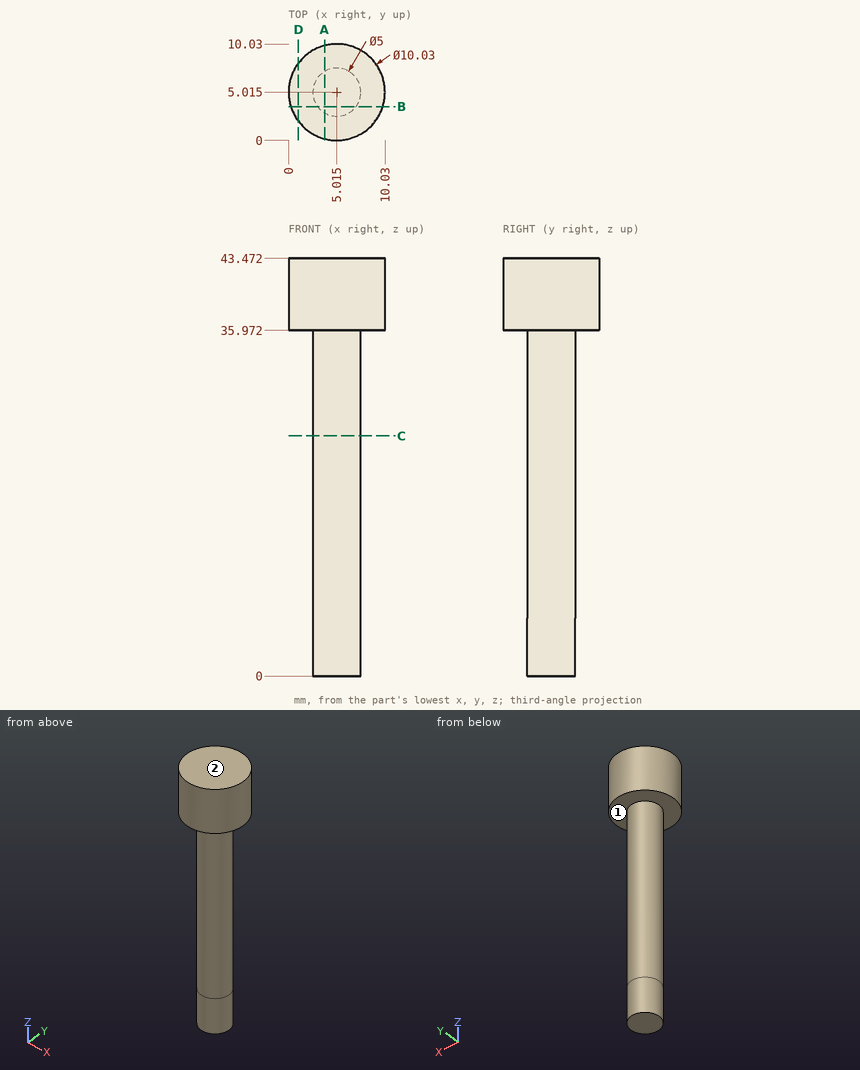
The figure shows three views and two pictorial views of one solid part (mm, origin at its lowest corner). Answer the questions. A direction names the side the tool comes from. Give positions to 0.01 mm unless a question says otherwise; leave off trailing zeros. Order: outer loops, then holes, each group sorted by start corner. A loop starts at its lowest first (then second) coordinate and runs counter-clockwise, first axis right, second up. Notation, with made-up numbers: (37.25, 16) -> (82.25, 16) arc R21 cw to (82.25, 32) -> close; hole circle Ø1 at (-29, 22.5). An arc over 180 degrees is marked (long way). Answer as a JSON object with one key per item and string values. Group by question number.
Item 1: Consider L1, parallel to Z at x = 9, y = 3.75; L2, parallel to Y at x = 4.5, z = 23; L3, parallel to Y at x = 6, z = 26.5. Determine where each line is inside the solid, lowest interval first. Write a range as from..to.
Item 2: The part is cut by section D-D on x = 1. Write down the section's boundary in (y, z).
Item 3: The part is cut by section A-A on x = 3.75. Write down the section's boundary in (y, z).
Item 4: Flat-ended cylindrical pins translate along their axes: pin 1 (1.5 mm diameter, centred on y = 2, z = 30.5, fed in from +X); pin 2 (4 mm diameter, centred on y = 8, z = 37.5, fed in from +X); pin 3 (6 mm diameter, centred on y = 2, z = 10, fed in from -X). Find the tip coordinate at first contact, or state that the pin passes through.
Item 5: A tool of negligible diameter and unlimited length cuts with its end or side. For the marked faces 1 and 2, from which of +Z, -Z, +X, -X, +Y, -Y can it reach the whole face along a straight path? Write none if from no direction.
Item 6: The part is cut by section C-C on z = 25. Write down the section's boundary in (x, y) (3 decimals), and give its area (3 significant figures).
Item 7: The part is cut by section B-B on y = 3.5. Write down the section's boundary in (x, z), and give its area (3 significant figures).
Result set:
{
 "1": {"L1": "35.97..43.47", "L2": "2.57..7.46", "L3": "2.72..7.31"},
 "2": {"outline": "(2.01, 35.97) -> (8.02, 35.97) -> (8.02, 43.47) -> (2.01, 43.47) -> close"},
 "3": {"outline": "(0.16, 35.97) -> (2.86, 35.97) -> (2.86, 0) -> (7.17, 0) -> (7.17, 35.97) -> (9.87, 35.97) -> (9.87, 43.47) -> (0.16, 43.47) -> close"},
 "4": {"pin 1": "x = 6.07", "pin 2": "x = 9.93", "pin 3": "x = 2.52"},
 "5": {"face 1": "-Z", "face 2": "+Z, +X, -X, +Y, -Y"},
 "6": {"outline": "circle Ø5 at (5.015, 5.015)", "area": "19.6 mm²"},
 "7": {"outline": "(0.23, 35.97) -> (3.03, 35.97) -> (3.03, 0) -> (7, 0) -> (7, 35.97) -> (9.8, 35.97) -> (9.8, 43.47) -> (0.23, 43.47) -> close", "area": "215 mm²"}
}
